Read the model definition and answer for the solid it produces. Units are mm, in the model's axes. A direction names the side the tool comes from. Coordinates: 2 decimals unless noted, no trailing zeros. Loops run counter-clockwise (first coordinate to the right, second up) from the corner with the lowest first, then second, coordinate; pieces in that order, holes last. Notation, with made-up numbers: (-40, -11) - (-7, -11) arc R23 cw to (-7, 21) - close; hole circle Ø2 at (68, 79.5). An arc over 180 degrees is marked (long way). Use CSV: the item, a comma, the result in double quotes.
```python
from build123d import *

# Parameters (mm, degrees)
F0_W      = 16
F0_H      = 16
F1_DEPTH  = 16
F2_R      = 2
F7_R      = 1.75
F9_DEPTH  = 1
F5_R      = 1.4939144971
F5_R_2    = 1.3959315932
F5_R_3    = 1.4557452585
F5_R_4    = 1.6299524928
F5_R_5    = 1.296089905
F10_DEPTH = 1
F4_R      = 1.75
F11_DEPTH = 1
F3_R      = 1.75
F12_DEPTH = 1
F8_R      = 1.2715772804
F8_R_2    = 1.246518745
F8_R_3    = 1.0985297942
F8_R_4    = 1.1545407094
F13_DEPTH = 1
F6_R      = 1.2445916632
F6_R_2    = 1.5020712319
F6_R_3    = 1.2709069935
F14_DEPTH = 1


with BuildPart() as f1:
    # F0 (on Front) → F1 (new body)
    with BuildSketch(Plane.XZ):
        Rectangle(F0_W, F0_H)
    extrude(amount=F1_DEPTH)

    # F2
    f2_edges = [f1.edges().sort_by_distance(p)[0] for p in [
        (8, -16, 0),
        (0, -16, 8),
        (0, -16, -8),
        (-8, -16, 0),
        (-8, 0, 0),
        (-8, -8, 8),
        (-8, -8, -8),
        (0, 0, 8),
        (8, -8, 8),
        (8, 0, 0),
        (0, 0, -8),
        (8, -8, -8),
    ]]
    fillet(f2_edges, radius=F2_R)

    # F7 (on face) → F9 (cut)
    with BuildSketch(Plane.YZ.offset(8)):
        with Locations((-11.8932482252, -0.7234399795)):
            Circle(F7_R)
        with Locations((-6.4081071032, -0.375177088)):
            Circle(F7_R)
        with BuildLine():
            ThreePointArc((-5.1369685637, -4.2931345864), (-7.9793834546, -2.9259734013), (-7.2731167994, -6))
            Line((-7.2731167994, -6), (-6.500820328, -6))
            ThreePointArc((-6.500820328, -6), (-5.5198073785, -5.3855494773), (-5.1369685637, -4.2931345864))
        make_face()
        with BuildLine():
            Line((-10.225043764, -6), (-13.3873214242, -6))
            ThreePointArc((-13.3873214242, -6), (-11.8061825941, -7), (-10.225043764, -6))
        make_face()
        with BuildLine():
            ThreePointArc((-10.225043764, -6), (-10.0989197331, -5.6343872054), (-10.0561825941, -5.25))
            ThreePointArc((-10.0561825941, -5.25), (-12.1905697995, -3.5427371391), (-13.3873214242, -6))
            Line((-13.3873214242, -6), (-10.225043764, -6))
        make_face()
        with Locations((-6.3210414721, 4.0651748088)):
            Circle(F7_R)
        with Locations((-12.1979774444, 4.1522404399)):
            Circle(F7_R)
    extrude(amount=-F9_DEPTH, mode=Mode.SUBTRACT)

    # F5 (on face) → F10 (cut)
    with BuildSketch(Plane(origin=(0, 0, 0), x_dir=(-1, 0, 0), z_dir=(0, 1, 0))):
        Circle(F5_R)
        with Locations((3.0504588503, -3.3979776781)):
            Circle(F5_R_2)
        with Locations((-2.701072488, 3.6476475652)):
            Circle(F5_R_3)
        with Locations((3.3380351961, 3.4319653641)):
            Circle(F5_R_4)
        with Locations((-3.0605429783, -2.7509303764)):
            Circle(F5_R_5)
    extrude(amount=-F10_DEPTH, mode=Mode.SUBTRACT)

    # F4 (on face) → F11 (cut)
    with BuildSketch(Plane(origin=(-8, 0, 0), x_dir=(0, -1, 0), z_dir=(-1, 0, 0))):
        with Locations((7.2365845554, 0)):
            Circle(F4_R)
    extrude(amount=-F11_DEPTH, mode=Mode.SUBTRACT)

    # F3 (on face) → F12 (cut)
    with BuildSketch(Plane.XZ.offset(16)):
        with Locations((-3.2950715739, -2.6576476197)):
            Circle(F3_R)
        with Locations((2.4981695437, 3.135593015)):
            Circle(F3_R)
    extrude(amount=-F12_DEPTH, mode=Mode.SUBTRACT)

    # F8 (on face) → F13 (cut)
    with BuildSketch(Plane(origin=(0, 0, -8), x_dir=(1, 0, 0), z_dir=(0, 0, -1))):
        with Locations((-3.9973538369, 11.7731597275)):
            Circle(F8_R)
        with Locations((2.0313244313, 11.7103606462)):
            Circle(F8_R_2)
        with Locations((-3.2437690534, 6.1840731651)):
            Circle(F8_R_3)
        with Locations((1.5289339935, 5.7444819249)):
            Circle(F8_R_4)
    extrude(amount=-F13_DEPTH, mode=Mode.SUBTRACT)

    # F6 (on face) → F14 (cut)
    with BuildSketch(Plane.XY.offset(8)):
        with Locations((-4.1440962814, -11.7570487782)):
            Circle(F6_R)
        with Locations((0, -8.6503596976)):
            Circle(F6_R_2)
        with Locations((3.5650942009, -5.1984833553)):
            Circle(F6_R_3)
    extrude(amount=-F14_DEPTH, mode=Mode.SUBTRACT)


solid = f1.part
```
Q1. For a pull along Y with two mould halves and no side action, classify faces 1 (the face through (-7.43, -0.6, 0.08)), 2 (the face through (-4.306, -10.523, 7.507)), 3 (the face through (-7.43, -8.08, -7.4)), 4 (the face through (-3, -15, -3)) as +Y half, -Y half, draft (parallel to the pull), parting line (faces both ways), or undercut.
Reported:
face 1,"+Y half"
face 2,"undercut"
face 3,"draft"
face 4,"-Y half"
Q2. The part is cut by section A-A on x = 0. Determine the outline of the cut face in (y, z).
Reported:
outline,"(-16, -6) arc R2 ccw to (-14, -8) - (-2, -8) arc R2 ccw to (0, -6) - (0, -1.49) - (-1, -1.49) - (-1, 1.49) - (0, 1.49) - (0, 6) arc R2 ccw to (-2, 8) - (-7.15, 8) - (-7.15, 7) - (-10.15, 7) - (-10.15, 8) - (-14, 8) arc R2 ccw to (-16, 6) - close"
Q3. The part is cut by section C-C on z = 0. Determine the outline of the cut face in (x, y), and give its area (3 significant figures).
Reported:
outline,"(-8, -14) arc R2 ccw to (-6, -16) - (6, -16) arc R2 ccw to (8, -14) - (8, -13.49) - (7, -13.49) - (7, -10.3) - (8, -10.3) - (8, -8.12) - (7, -8.12) - (7, -4.7) - (8, -4.7) - (8, -2) arc R2 ccw to (6, 0) - (1.49, 0) - (1.49, -1) - (-1.49, -1) - (-1.49, 0) - (-6, 0) arc R2 ccw to (-8, -2) - (-8, -5.49) - (-7, -5.49) - (-7, -8.99) - (-8, -8.99) - close"
area,"239 mm²"
Q4. Find the intervals of material crossed by probe 1 along Z at (x, y) = (3.25, -5); probe 2 along Z at (x, y) = (2, -6), in increasing order. Write a range as [from, to].
Reported:
probe 1,"z = [-8, 7]"
probe 2,"z = [-7, 8]"
Q5. The part is cut by section B-B on y = -1.5. Determine the outline of the cut face in (x, z).
Reported:
outline,"(-7.94, -6) arc R1.94 ccw to (-6, -7.94) - (6, -7.94) arc R1.94 ccw to (7.94, -6) - (7.94, 6) arc R1.94 ccw to (6, 7.94) - (-6, 7.94) arc R1.94 ccw to (-7.94, 6) - close"
Q6. A tool of negligible diameter and unlimited length cuts with its end or side. For faces 5 (the face through (4, -5, 7)), 6 (the face through (7.51, -5.38, 5.54)), 7 (the face through (4.355, -0.493, -2.694)), 8 (the face through (-3.314, -12.845, -7.507)), from which of +Z, -Z, +X, -X, +Y, -Y can it reach the whole face along a straight path? Write none if from no direction.
Reported:
face 5,"+Z"
face 6,"+X"
face 7,"+Y"
face 8,"-Z"
Q7. Given P1, Ø0.7, axis at x = 2, y = -12, coming from the -Z side; P2, Ø0.7, axis at x = -4.5, y = -11, coming from the +Z side; P3, Ø2, axis at y = -6.41, z = -0.38, coming from the +X side, each flat-ended and moving along its own axis, determine where each tip first touches the part or whether it passes through.
Reported:
P1,"stops at z = -7"
P2,"stops at z = 7"
P3,"stops at x = 7"
